Here's how the part is built. I have some questions about the finished solid (model axes, mm). Round coordinates to 2 decimals unless told otherwise and drop trailing zeros. Write each loop counter-clockwise with the first axis right and the second up, starting at its lowest first coordinate (ties: lowest second). Pieces come first, ordered by that corner, then holes. Notation, with made-up numbers: M -27.5,52 L 0.5,52 A14 ccw 0.5,57 Z; hole C 29.5,44.5 d6. An arc over 180 degrees is marked long. Write item = value, one per line. Start each with the question number.
(1) I need wall thicknesses on line 1 along Z through (x, y) = (0, 2.25) (3 decimals); line 2 along X through (y, z) = (-0.75, -22.5); line 3 along X through (y, z) = (-2.5, -27.5). Which ranges of each line are inside material? Lowest first, please.
(2) I want a section at A-A (z = -27). List the corners of the cut face in (x, y) for me (3 decimals).
(3) I want a section at B-B (y = 0). List the corners of the cut face in (x, z) for me, and give its area (3 significant figures).
(4) I want a section at D-D (z = 6). List the corners of the cut face in (x, y) for me (3 decimals), and give its area (3 significant figures).
(5) I want a section at C-C (x = 0). List the corners of the cut face in (y, z) for me (3 decimals).
(6) Will these pins go through, and if not, where does the flat tip stop? pin 1 Ø21 at (x, z) = (-18, 14.5) entering from -Y (3 decimals); pin 2 Ø0.8 at (x, y) = (20, -1) entering from -Z; pin 3 Ø3 at (y, z) = (1, 30) entering from +X; pin 4 Ø1.5 at (y, z) = (2.5, 22.5) entering from -X.
```python
from build123d import *

# Parameters (mm, degrees)
F0_R     = 2.3876
F0_W     = 11.9644477963
F0_H     = 25.4
F0_W_2   = 2.794
F0_H_2   = 18.8976
F1_DEPTH = 3.175
F3_W     = 2.54
F3_H     = 25.4
F4_DEPTH = 2.54
F6_W     = 2.54
F6_H     = 25.4
F7_DEPTH = 2.54


with BuildPart() as f1:
    # F0 (on Front) → F1 (new body, symmetric)
    with BuildSketch(Plane.XZ):
        with BuildLine():
            Line((-9.4017383467, 23.2221963037), (-31.0533456504, 0))
            ThreePointArc((-31.0533456504, 0), (1.5738401562, -75.0292582617), (34.2010259628, 0))
            Line((34.2010259628, 0), (12.5494186591, 23.2221963037))
            Line((12.5494186591, 23.2221963037), (12.5494186591, 43.8596963037))
            Line((12.5494186591, 43.8596963037), (-9.4017383467, 43.8596963037))
            Line((-9.4017383467, 43.8596963037), (-9.4017383467, 23.2221963037))
        make_face()
        with Locations((0, -54.2525947094)):
            Circle(F0_R, mode=Mode.SUBTRACT)
        with Locations((0, -25.0313151628)):
            Rectangle(F0_W, F0_H, mode=Mode.SUBTRACT)
        with Locations((19.9750838982, -28.2825151628)):
            Rectangle(F0_W_2, F0_H_2, mode=Mode.SUBTRACT)
        with Locations((0, 10.739565827)):
            Circle(F0_R, mode=Mode.SUBTRACT)
    extrude(amount=F1_DEPTH, both=True)

    # F3 (on offset) → F4 (cut)
    with BuildSketch(Plane(origin=(-16.6122141895, 0, 15.4886787354), x_dir=(0, -1, 0), z_dir=(-0.7314077576, 0, 0.6819403875))):
        with Locations((0, -4.733831039)):
            Rectangle(F3_W, F3_H)
    extrude(amount=-F4_DEPTH, mode=Mode.SUBTRACT)

    # F6 (on offset) → F7 (cut)
    with BuildSketch(Plane(origin=(18.2960887755, 0, 17.0586676721), x_dir=(0, 1, 0), z_dir=(0.7314077576, 0, 0.6819403875))):
        with Locations((0, -6.8803708986)):
            Rectangle(F6_W, F6_H)
    extrude(amount=-F7_DEPTH, mode=Mode.SUBTRACT)


solid = f1.part
```
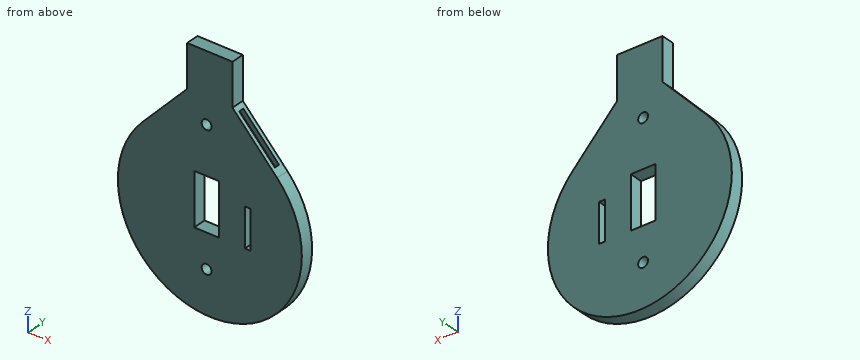
Returned:
q1.line_1 = -75.001 to -56.64, -51.865 to -37.731, -12.331 to 8.352, 13.127 to 43.86
q1.line_2 = -42.33 to -5.98, 5.98 to 18.58, 21.37 to 45.47
q1.line_3 = -42.94 to -5.98, 5.98 to 18.58, 21.37 to 46.09
q2.outline = M -42.904,-3.175 L -5.982,-3.175 L -5.982,3.175 L -42.904,3.175 Z; M 5.982,-3.175 L 18.578,-3.175 L 18.578,3.175 L 5.982,3.175 Z; M 21.372,-3.175 L 46.051,-3.175 L 46.051,3.175 L 21.372,3.175 Z
q3.outline = M -31.05,0 A44.61 ccw long 34.2,0 L 31.65,2.74 L 29.79,1.01 L 12.47,19.58 L 14.33,21.32 L 12.55,23.22 L 12.55,43.86 L -9.4,43.86 L -9.4,23.22 L -11.18,21.32 L -9.32,19.58 L -26.64,1.01 L -28.5,2.74 Z; hole M -5.98,-37.73 L 5.98,-37.73 L 5.98,-12.33 L -5.98,-12.33 Z; hole C 0,-54.25 d4.78; hole C 0,10.74 d4.78; hole M 18.58,-37.73 L 21.37,-37.73 L 21.37,-18.83 L 18.58,-18.83 Z
q3.area = 6,560 mm²
q4.outline = M -25.459,-3.175 L 28.607,-3.175 L 28.607,-1.27 L 25.134,-1.27 L 25.134,1.27 L 28.607,1.27 L 28.607,3.175 L -25.459,3.175 L -25.459,1.27 L -21.986,1.27 L -21.986,-1.27 L -25.459,-1.27 Z
q4.area = 326 mm²
q5.outline = M -3.175,-75.001 L 3.175,-75.001 L 3.175,-56.64 L -3.175,-56.64 Z; M -3.175,-51.865 L 3.175,-51.865 L 3.175,-37.731 L -3.175,-37.731 Z; M -3.175,-12.331 L 3.175,-12.331 L 3.175,8.352 L -3.175,8.352 Z; M -3.175,13.127 L 3.175,13.127 L 3.175,43.86 L -3.175,43.86 Z
q6.pin_1 = -3.175
q6.pin_2 = -71.22
q6.pin_3 = 12.55
q6.pin_4 = -10.77
